Source: CAD feature listing. Evaluate the final solid. Frame: model axes, mm. Face numbers are marked on the shaded views. A direction names the side the tool comes from. Round coordinates to 2 decimals unless told otherwise and drop trailing zeros. Order: outer loops, then holes, each group sorted by start corner. A loop starts at its lowest first (then second) coordinate and runs counter-clockwise, first axis right, second up. Notation, with made-up numbers: (18, -9.5) -> (60, -9.5) arc R16 cw to (60, 11.5) -> close; hole circle Ø9 at (-14, 57.5). An arc over 180 degrees is marked (long way). Write item = value, one per line. Start each with the question number.
(1) Cut plane B-B on z = 12.7. Return the cut outline in (x, y) (3 decimals), then the cut area to 3 significant figures.
(2) Ray query, line 1 (Y direction, x = 11.25, z = 5) (3 decimals); line 2 (Y direction, x = 1.45, z = 38.1); line 3 (X direction, y = 29, z = 24) (3 decimals). Return the intervals inside material, ascending.
(3) Cut plane D-D on y = 15. Return the cut outline in (x, z) (3 decimals).
(4) Cut plane A-A on x = 13.75. Return the cut outline in (y, z) (3 decimals), then the cut area to 3 significant figures.
(5) Draft query along X for the marked faces 1, 2 and 3. Return one class per face: released by +X, released by -X, zero draft, split by the parting line, or undercut.
(6) Cut plane C-C on y = 38.1. Return the cut outline in (x, z) (3 decimals).
(7) Reachability of the marked faces 4 and 5 from +Z, -Z, +X, -X, +Y, -Y: full face, straight path, thin tool, end or side. Return the list, or none.
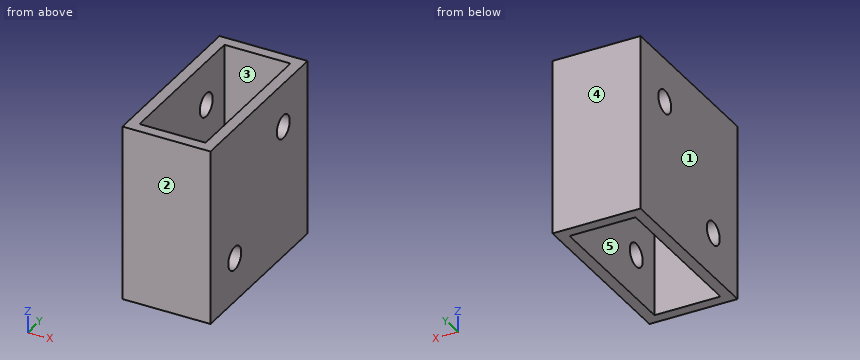
Autodesk Inventor part; units mm, degrees
ref_plane "YZ Plane" through (0, 0, 0) normal (1, 0, 0) x (0, 1, 0)
ref_plane "XZ Plane" through (0, 0, 0) normal (0, 1, 0) x (-1, 0, 0)
ref_plane "XY Plane" through (0, 0, 0) normal (0, 0, 1) x (1, 0, 0)
sketch "Sketch1" plane through (0, 0, 0) normal (0, 0, 1) x (1, 0, 0)
  line L0 (0, 0) -> (25.4, 0)
  line L1 (25.4, 0) -> (25.4, 50.8)
  line L2 (25.4, 50.8) -> (0, 50.8)
  line L3 (0, 50.8) -> (0, 0)
  line L4 (3.175, 3.175) -> (22.225, 3.175)
  line L5 (22.225, 3.175) -> (22.225, 47.625)
  line L6 (22.225, 47.625) -> (3.175, 47.625)
  line L7 (3.175, 47.625) -> (3.175, 3.175)
  dimension "d0" = 25.4
  dimension "d1" = 50.8
  dimension "d2" = 3.175
extrude "Extrusion1" add sketch "Sketch1" along normal blind 50.8
sketch "Sketch2" plane through (25.4, 0, 0) normal (1, 0, 0) x (0, 0, -1)
  circle A0 centre (-38.1, 38.1) radius 3.3734
  circle A1 centre (-12.7, 12.7) radius 3.3734
  line L0 (-50.8, 0) -> (-50.8, 50.8)
  line L1 (0, 50.8) -> (-50.8, 50.8)
  line L2 (0, 0) -> (0, 50.8)
  line L3 (0, 0) -> (-50.8, 0)
  dimension "d5" = 6.7469
  dimension "d6" = 6.7469
  dimension "d7" = 12.7
  dimension "d8" = 12.7
  dimension "d9" = 12.7
  dimension "d10" = 12.7
extrude "Extrusion2" cut sketch "Sketch2" against normal blind 25.4 contours A0 | A1
properties part number "2nd flywheel block"
Evaluation:
q1.outline = (0, 0) -> (25.4, 0) -> (25.4, 9.327) -> (22.225, 9.327) -> (22.225, 3.175) -> (3.175, 3.175) -> (3.175, 9.327) -> (0, 9.327) -> close; (0, 16.073) -> (3.175, 16.073) -> (3.175, 47.625) -> (22.225, 47.625) -> (22.225, 16.073) -> (25.4, 16.073) -> (25.4, 50.8) -> (0, 50.8) -> close
q1.area = 401 mm^2
q2.line_1 = 0 to 3.175, 47.625 to 50.8
q2.line_2 = 0 to 34.73, 41.47 to 50.8
q2.line_3 = 0 to 3.175, 22.225 to 25.4
q3.outline = (0, 0) -> (3.175, 0) -> (3.175, 10.232) -> (0, 10.232) -> close; (0, 15.168) -> (3.175, 15.168) -> (3.175, 50.8) -> (0, 50.8) -> close; (22.225, 0) -> (25.4, 0) -> (25.4, 10.232) -> (22.225, 10.232) -> close; (22.225, 15.168) -> (25.4, 15.168) -> (25.4, 50.8) -> (22.225, 50.8) -> close
q4.outline = (0, 0) -> (3.175, 0) -> (3.175, 50.8) -> (0, 50.8) -> close; (47.625, 0) -> (50.8, 0) -> (50.8, 50.8) -> (47.625, 50.8) -> close
q4.area = 323 mm^2
q5.face_1 = released by -X
q5.face_2 = zero draft
q5.face_3 = undercut
q6.outline = (0, 0) -> (3.175, 0) -> (3.175, 34.727) -> (0, 34.727) -> close; (0, 41.473) -> (3.175, 41.473) -> (3.175, 50.8) -> (0, 50.8) -> close; (22.225, 0) -> (25.4, 0) -> (25.4, 34.727) -> (22.225, 34.727) -> close; (22.225, 41.473) -> (25.4, 41.473) -> (25.4, 50.8) -> (22.225, 50.8) -> close
q7.face_4 = +Z, -Z, +X, -X, +Y
q7.face_5 = +Z, -Z
